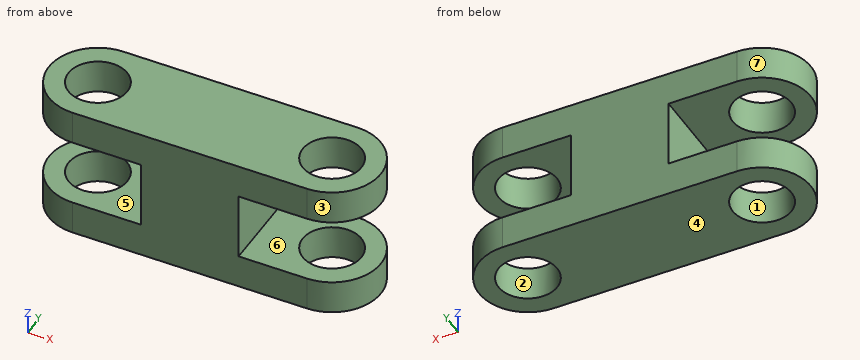
Autodesk Inventor part; units mm, degrees
ref_plane "YZ Plane" through (0, 0, 0) normal (1, 0, 0) x (0, 1, 0)
ref_plane "XZ Plane" through (0, 0, 0) normal (0, 1, 0) x (-1, 0, 0)
ref_plane "XY Plane" through (0, 0, 0) normal (0, 0, 1) x (1, 0, 0)
sketch "草图1" plane through (0, 0, 0) normal (0, 0, 1) x (1, 0, 0)
  line L0 (-44.0519, -22.2048) -> (24.7481, -22.2048)
  line L1 (-44.0519, -22.2048) -> (-44.0519, 41.5952)
  line L2 (-104.0519, 2.7952) -> (15.9481, 2.7952)
  line L3 (15.9481, -47.2048) -> (-104.0519, -47.2048)
  line L4 (-104.0519, 2.7952) -> (15.9481, -47.2048) construction
  line L5 (15.9481, 2.7952) -> (-104.0519, -47.2048) construction
  arc A0 (15.9481, -47.2048) -> (15.9481, 2.7952) centre (15.9481, -22.2048) ccw
  arc A1 (-104.0519, 2.7952) -> (-104.0519, -47.2048) centre (-104.0519, -22.2048) ccw
  circle A2 centre (-104.0519, -22.2048) radius 15
  circle A3 centre (15.9481, -22.2048) radius 15
  dimension "d2" = 25
  dimension "d3" = 50
  dimension "d4" = 120
  dimension "d7" = 30
  dimension "d8" = 30
  dimension "d14" = 50
extrude "拉伸1" add sketch "草图1" along normal blind 70
sketch "草图2" plane through (-104.0519, 2.7952, 0) normal (0, 1, 0) x (1, 0, 0)
  line L0 (0, 0) -> (120, 0)
  line L1 (60, 0) -> (60, -70)
  line L2 (120, -70) -> (0, -70)
  line L3 (-25, 0) -> (-25, -70)
  line L4 (-25, -35) -> (145, -35)
  line L5 (145, 0) -> (145, -70)
  line L6 (145, -17.5) -> (145, -52.5)
  line L7 (-25, -52.5) -> (-25, -17.5)
  line L8 (-25, -17.5) -> (145, -52.5) construction
  line L9 (145, -17.5) -> (-25, -52.5) construction
  line L10 (35, -17.5) -> (35, -52.5)
  line L11 (85, -17.5) -> (85, -52.5)
  line L12 (145, -52.5) -> (85, -52.5)
  line L13 (35, -52.5) -> (-25, -52.5)
  line L14 (-25, -17.5) -> (35, -17.5)
  line L15 (85, -17.5) -> (145, -17.5)
  point P0 (104.0519, 0)
  point P1 (60, -35)
  dimension "d10" = 60
  dimension "d11" = 60
  dimension "d15" = 35
  dimension "d16" = 17.5
  dimension "d17" = 35
extrude "拉伸2" cut sketch "草图2" against normal blind 70
properties part number "ConnectBoard" material "钢，高强度，低合金"
Geometry: final body of the model. Coordinates: model frame, mm. Face numbers are marked on the shaded views. A direction names the side the tool comes from. Give positions to 0.01 mm unless a question says otherwise; leave off trailing zeros. Loops run counter-clockwise (first coordinate to the right, second up) from the corner with the lowest first, then second, coordinate; pieces in that order, holes last. Notation, with made-up numbers: (-36.75, -9.5) - (-11.75, -9.5) arc R31 ccw to (-11.75, 22.5) - close; hole circle Ø8 at (22, 19.25). An arc over 180 degrees is marked (long way). One line per question, with ' | ' between items. Start each with the question number.
(1) Section query C-C on z = 14. Return loops of the section in (x, y), then the cut area to 3 significant figures.
(2) Contact query for flat-ended pins moving along their axis: pin 1 (10 mm diameter, centred on y = -37, z = 54.5, fed in from -X); pin 2 (8 mm diameter, centred on y = -26.5, z = 45.5, fed in from -X); pin 3 (1 mm diameter, centred on x = 24, y = -33, fed in from +Z). Output: stop coordinate, or through.
(3) Reachability of the marked faces 5, 6 and 7 from +Z, -Z, +X, -X, +Y, -Y: full face, straight path, thin tool, end or side. Return the list, or none.
(4) Section query B-B on x = -73. Return loops of the section in (y, z).
(5) Ray query, line 1 (Z direction, x = -16.5, y = -16); line 2 (X direction, y = -18, z = 14); line 3 (X direction, y = -35, z = 38). Return the intervals inside material, ascending. Write a range as from..to.
(6) Section query A-A on y = -12. Return loops of the section in (x, z).
(7) Section query D-D on x = 7.5. Return loops of the section in (y, z).
(8) Pull-direction query (Y, two-part tool) for the marked faces 1, 2, 3 and 4; classes: released by +Y, released by -Y, zero draft, split by the parting line, or undercut.
The answers:
1) outline: (-104.05, -47.2) - (15.95, -47.2) arc R25 ccw to (15.95, 2.8) - (-104.05, 2.8) arc R25 ccw to start; hole circle Ø30 at (-104.05, -22.2); hole circle Ø30 at (15.95, -22.2) | area: 6,550 mm2
2) pin 1: x = -127.05 | pin 2: x = -69.05 | pin 3: through
3) face 5: -X, +Y, -Y | face 6: +X, +Y, -Y | face 7: +Z, -Z, -X
4) outline: (-47.2, 0) - (2.8, 0) - (2.8, 17.5) - (-47.2, 17.5) - close; (-47.2, 52.5) - (2.8, 52.5) - (2.8, 70) - (-47.2, 70) - close
5) line 1: 0..17.5, 52.5..70 | line 2: -128.7..-118.45, -89.65..1.55, 30.35..40.59 | line 3: -69.05..-19.05
6) outline: (-126.87, 0) - (-115.05, 0) - (-115.05, 17.5) - (-126.87, 17.5) - close; (-126.87, 52.5) - (-115.05, 52.5) - (-115.05, 70) - (-126.87, 70) - close; (-93.06, 0) - (4.95, 0) - (4.95, 17.5) - (-19.05, 17.5) - (-19.05, 52.5) - (4.95, 52.5) - (4.95, 70) - (-93.06, 70) - (-93.06, 52.5) - (-69.05, 52.5) - (-69.05, 17.5) - (-93.06, 17.5) - close; (26.94, 0) - (38.77, 0) - (38.77, 17.5) - (26.94, 17.5) - close; (26.94, 52.5) - (38.77, 52.5) - (38.77, 70) - (26.94, 70) - close
7) outline: (-47.2, 0) - (-34.6, 0) - (-34.6, 17.5) - (-47.2, 17.5) - close; (-47.2, 52.5) - (-34.6, 52.5) - (-34.6, 70) - (-47.2, 70) - close; (-9.81, 0) - (2.8, 0) - (2.8, 17.5) - (-9.81, 17.5) - close; (-9.81, 52.5) - (2.8, 52.5) - (2.8, 70) - (-9.81, 70) - close
8) face 1: undercut | face 2: undercut | face 3: split by the parting line | face 4: zero draft
